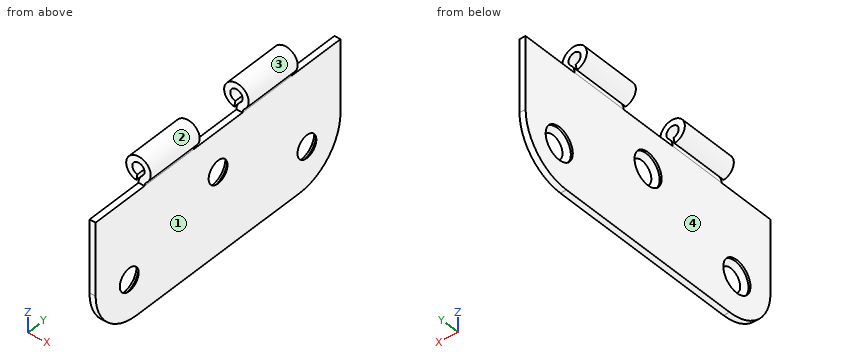
```python
from build123d import *

# Parameters (mm, degrees)
BOSS_EXTRUDE1_DEPTH                       = 38.1
SKETCH3_W                                 = 6.724757914
SKETCH3_H                                 = 15.24
CUT_EXTRUDE1_DEPTH                        = 4.175
CUT_EXTRUDE1_DEPTH_BACK                   = 4.175
CSK_FOR_8_FLAT_HEAD_MACHINE_SCREW_2_COUNT = 2
CSK_FOR_8_FLAT_HEAD_MACHINE_SCREW_2_PITCH = 29.553945574
CSK_FOR_8_FLAT_HEAD_MACHINE_SCREW_3_COUNT = 2
CSK_FOR_8_FLAT_HEAD_MACHINE_SCREW_3_PITCH = 55.283171943
FILLET1_R                                 = 12.7


with BuildPart() as part:
    # Sketch2 → Boss-Extrude1 (new body, symmetric)
    with BuildSketch(Plane(origin=(0, 0, 0), x_dir=(1, 0, 0), z_dir=(0, 1, 0))):
        with BuildLine():
            Line((1.5875, 34.925), (0, 34.925))
            Line((0, 34.925), (0, 3.549757914))
            ThreePointArc((0, 3.549757914), (0.2766348, 2.253569592), (1.058333333, 1.183252638))
            ThreePointArc((1.058333333, 1.183252638), (-0.435047689, -1.526725175), (-0.275666482, 1.563382308))
            Line((-0.275666482, 1.563382308), (-0.551332964, 3.126764616))
            ThreePointArc((-0.551332964, 3.126764616), (-0.870095378, -3.053450349), (2.116666667, 2.366505276))
            ThreePointArc((2.116666667, 2.366505276), (1.7258174, 2.901663753), (1.5875, 3.549757914))
            Line((1.5875, 3.549757914), (1.5875, 34.925))
        make_face()
    extrude(amount=BOSS_EXTRUDE1_DEPTH, both=True)

    # Sketch3 → Cut-Extrude1 (cut, two sides)
    with BuildSketch(Plane(origin=(0, 0, 0), x_dir=(0, 0, -1), z_dir=(1, 0, 0))) as cut_extrude1_sk:
        with Locations((0.187378957, 30.48)):
            Rectangle(SKETCH3_W, SKETCH3_H)
        with Locations((0.187378957, 0)):
            Rectangle(SKETCH3_W, SKETCH3_H)
        with Locations((0.187378957, -30.48)):
            Rectangle(SKETCH3_W, SKETCH3_H)
    extrude(amount=CUT_EXTRUDE1_DEPTH, mode=Mode.SUBTRACT)
    extrude(cut_extrude1_sk.sketch, amount=-CUT_EXTRUDE1_DEPTH_BACK, mode=Mode.SUBTRACT)

    # Sketch4 → CSK for #8 Flat Head Machine Screw (100)1 (revolve, cut)
    with BuildSketch(Plane(origin=(0, -27.641585971, -24.466585971), x_dir=(0, 0, 1), z_dir=(0, 1, 0))):
        Polygon((0, 0), (0, 3.175), (2.2479, 3.175), (2.2479, 2.159767624), (4.2164, 0.508), (4.2164, 0), align=None)
    csk_for_8_flat_head_machine_screw_100 = revolve(axis=Axis((-6.35, -27.641585971, -24.466585971), (1, 0, 0)), mode=Mode.SUBTRACT)

    # CSK for _8 Flat Head Machine Screw _ 2: CSK for #8 Flat Head Machine Screw (100)1 ×2
    with Locations(*[Vector(0, 0.935292579, 0.35387539) * (i * CSK_FOR_8_FLAT_HEAD_MACHINE_SCREW_2_PITCH) for i in range(1, CSK_FOR_8_FLAT_HEAD_MACHINE_SCREW_2_COUNT)]):
        add(csk_for_8_flat_head_machine_screw_100, mode=Mode.SUBTRACT)

    # CSK for _8 Flat Head Machine Screw _ 3: CSK for #8 Flat Head Machine Screw (100)1 ×2
    with Locations(*[(0, i * CSK_FOR_8_FLAT_HEAD_MACHINE_SCREW_3_PITCH, 0) for i in range(1, CSK_FOR_8_FLAT_HEAD_MACHINE_SCREW_3_COUNT)]):
        add(csk_for_8_flat_head_machine_screw_100, mode=Mode.SUBTRACT)

    # Fillet1
    fillet1_edges = [part.edges().sort_by_distance(p)[0] for p in [
        (0.79375, 38.1, -34.925),
        (0.79375, -38.1, -34.925),
    ]]
    fillet(fillet1_edges, radius=FILLET1_R)


solid = part.part
```
Geometry check sheet. Reference: the model listing, model coordinates, mm. Face numbers are marked on the shaded views. A direction names the side the tool comes from. Coordinates: 2 decimals unless noted, no trailing zeros. Write each loop counter-clockwise with the first axis right and the second up, starting at its lowest first coordinate (ties: lowest second). Pieces come first, ordered by that corner, then holes. Notation, with made-up numbers: M 14,29.25 L 48,29.25 A17 ccw 48,50.25 Z; hole C -38.75,-12 d6. An arc over 180 degrees is marked long. Answer as a JSON object with one key per item and string values.
1. Tool access check on the marked faces 3 and 4. Record the directions out of +Z, -Z, +X, -X, +Y, -Y that give a thin tool (end or side, any length) a straight path to the whole face; none if there is none.
Answers below:
{"face 3": "+Y, -Y", "face 4": "-Z, -X, +Y, -Y"}
2. Section check A-A, the plane z = 0. Enter the section's corners in (x, y) (1 decimal), plus the area to 3 significant figures.
Answers below:
{"outline": "M -3.2,-22.9 L -1.6,-22.9 L -1.6,-7.6 L -3.2,-7.6 Z; M -3.2,7.6 L -1.6,7.6 L -1.6,22.9 L -3.2,22.9 Z; M 1.6,-22.9 L 3.2,-22.9 L 3.2,-7.6 L 1.6,-7.6 Z; M 1.6,7.6 L 3.2,7.6 L 3.2,22.9 L 1.6,22.9 Z", "area": "96.8 mm²"}
3. Section check B-B, the plane y = 0. Enter the section's corners in (x, z) (1 decimal).
Answers below:
{"outline": "M 0,-34.9 L 1.6,-34.9 L 1.6,-16.9 L 0.5,-18.2 L 0,-18.2 Z; M 0,-9.8 L 0.5,-9.8 L 1.6,-11.1 L 1.6,-3.5 L 0,-3.5 Z"}
4. Go/stop test with flat-tipped pins: pin 1 Ø2.5 at (x, z) = (0, 0) entering from +Y; pin 2 Ø5 at (y, z) = (-9.5, -5.5) entering from +X; pin 3 Ø11 at (y, z) = (0, -14.01) entering from +X; pin 4 Ø1.7 at (x, y) = (0.5, 28.5) entering from +Z. Record where each tip stops, or that it passes through.
Answers below:
{"pin 1": "passes through", "pin 2": "stops at x = 1.69", "pin 3": "stops at x = 1.59", "pin 4": "stops at z = -3.55"}
5. Section check D-D, the plane z = -8.5. Enter the section's corners in (x, y), plus the area to 3 significant figures.
Answers below:
{"outline": "M 0,-38.1 L 1.59,-38.1 L 1.59,38.1 L 0,38.1 Z", "area": "121 mm²"}
6. Scan lines: L1, parallel to Y at x = 1.75, z = 0; L2, parallel to X at y = -18.25, z = 0 (1 decimal); L3, parallel to Z at x = 1.5, y = 24 (3 decimals). Record each from-to range of solid material in increasing order.
Answers below:
{"L1": "y = -22.86 to -7.62, 7.62 to 22.86", "L2": "x = -3.2 to -1.6, 1.6 to 3.2", "L3": "z = -34.925 to -3.55"}
7. Draft check along Z on the marked faces 1 and 2. Enter one of: released by +Z, released by -Z, zero draft, split by the parting line, or undercut.
Answers below:
{"face 1": "zero draft", "face 2": "split by the parting line"}
8. Section check C-C, the plane z = -23. Give the number of separate pieces and of enclosed holes in the cut face, plus the area to 3 significant figures.
Answers below:
{"separate pieces": "3", "enclosed holes": "0", "area": "98.8 mm²"}
